Check sheet for the modelled part. Datum: model origin and axes. Units: mm. A direction names the side the tool comes from. Coordinates: 2 decimals unless noted, no trailing zeros. Loops run counter-clockwise (first coordinate to the right, second up) from the corner with the lowest first, then second, coordinate; pieces in that order, holes last. Notation, with made-up numbers: M -10,36 L 45,36 A19 cw 45,65 Z; hole C 1.5,-37.5 d5. An arc over 180 degrees is marked long. Return JSON: item names as keys, results as strings.
from build123d import *

# Parameters (mm, degrees)
BOSS_EXTRUDE1_DEPTH = 145.0848
SKETCH2_R           = 4.50215
SKETCH2_W           = 12.192
SKETCH2_H           = 13.1191
CUT_EXTRUDE1_DEPTH  = 6.35
SKETCH3_W           = 13.1064
SKETCH3_H           = 5.9944
CUT_EXTRUDE2_DEPTH  = 6.35
SKETCH4_W           = 13.0429
SKETCH4_H           = 5.9944
CUT_EXTRUDE3_DEPTH  = 6.35


with BuildPart() as part:
    # Sketch1 → Boss-Extrude1 (new body)
    with BuildSketch(Plane.XY):
        with BuildLine():
            Line((3.110233801, 25.508957203), (61.149233801, 12.137799255))
            ThreePointArc((61.149233801, 12.137799255), (62.566459918, 11.24428163), (63.119, 9.662635945))
            Line((63.119, 9.662635945), (63.119, 2.54))
            ThreePointArc((63.119, 2.54), (62.375051224, 0.743948776), (60.579, 0))
            Line((60.579, 0), (2.54, 0))
            ThreePointArc((2.54, 0), (0.743948776, 0.743948776), (0, 2.54))
            Line((0, 2.54), (0, 23.033793893))
            ThreePointArc((0, 23.033793893), (0.958354315, 25.021253811), (3.110233801, 25.508957203))
        make_face()
    extrude(amount=BOSS_EXTRUDE1_DEPTH)

    # Sketch2 → Cut-Extrude1 (cut)
    with BuildSketch(Plane.XY.offset(145.0848)):
        with Locations((38.989, 8.9154)):
            Circle(SKETCH2_R)
        with Locations((16.9164, 12.65555)):
            Rectangle(SKETCH2_W, SKETCH2_H)
    extrude(amount=-CUT_EXTRUDE1_DEPTH, mode=Mode.SUBTRACT)

    # Sketch3 → Cut-Extrude2 (cut)
    with BuildSketch(Plane.ZY):
        with Locations((31.9532, 10.1854)):
            Rectangle(SKETCH3_W, SKETCH3_H)
        with Locations((53.0352, 10.1854)):
            Rectangle(SKETCH3_W, SKETCH3_H)
        with Locations((74.1172, 10.1854)):
            Rectangle(SKETCH3_W, SKETCH3_H)
        with Locations((95.1992, 10.1854)):
            Rectangle(SKETCH3_W, SKETCH3_H)
        with Locations((116.2812, 10.1854)):
            Rectangle(SKETCH3_W, SKETCH3_H)
    extrude(amount=-CUT_EXTRUDE2_DEPTH, mode=Mode.SUBTRACT)

    # Sketch4 → Cut-Extrude3 (cut)
    with BuildSketch(Plane(origin=(0, 0, 0), x_dir=(-1, 0, 0), z_dir=(0, 0, -1))):
        with Locations((-13.68425, 10.1981)):
            Rectangle(SKETCH4_W, SKETCH4_H)
        with Locations((-35.02025, 10.1981)):
            Rectangle(SKETCH4_W, SKETCH4_H)
    extrude(amount=-CUT_EXTRUDE3_DEPTH, mode=Mode.SUBTRACT)


solid = part.part
1) Draft check along Z on faces 1 (the face through (10.82, 13, 142)), 2 (the face through (25, 10, 0)), 3 (the face through (3, 10, 67.564)). Enter one of: +Z half, -Z half, draft (parallel to the pull), parting line (faces both ways), or undercut.
Answers:
{"face 1": "draft", "face 2": "-Z half", "face 3": "undercut"}
2) Section check A-A on z = 13. Record the cut outline in (x, y).
Answers:
{"outline": "M 0,2.54 A2.54 ccw 2.54,0 L 60.58,0 A2.54 ccw 63.12,2.54 L 63.12,9.66 A2.54 ccw 61.15,12.14 L 3.11,25.51 A2.54 ccw 0,23.03 Z"}
3) Scan lines: line 1 along Y through (x, z) = (3.5, 24); line 2 along X through (y, z) = (7.25, 99); line 3 along X through (y, z) = (5, 139.5). Record each from-to range of solid material in increasing order. Write a range as [from, to].
Answers:
{"line 1": "[0, 25.42]", "line 2": "[6.35, 63.12]", "line 3": "[0, 36.77], [41.21, 63.12]"}
4) Section check C-C on x = 13. Record the cut outline in (y, z).
Answers:
{"outline": "M 0,0 L 7.2,0 L 7.2,6.35 L 13.2,6.35 L 13.2,0 L 23.23,0 L 23.23,145.08 L 19.22,145.08 L 19.22,138.73 L 6.1,138.73 L 6.1,145.08 L 0,145.08 Z"}
5) Section check B-B on y = 14.75. Record the cut outline in (x, z).
Answers:
{"outline": "M 0,0 L 49.81,0 L 49.81,145.08 L 23.01,145.08 L 23.01,138.73 L 10.82,138.73 L 10.82,145.08 L 0,145.08 Z"}
6) Go/stop test with flat-tipped pins: pin 1 Ø5 at (x, z) = (4, 52.5) entering from +Y; pin 2 Ø3 at (x, z) = (4.5, 93) entering from +Y; pin 3 Ø3 at (y, z) = (11, 76.5) entering from -X. Record where each tip stops, or that it passes through.
Answers:
{"pin 1": "y = 25.57", "pin 2": "y = 25.53", "pin 3": "x = 6.35"}
7) Set-up check for faces 4 (the face through (3, 7.188, 74)), 5 (the face through (23.012, 13, 142)), 6 (the face through (14, 13.195, 3)): record each of +Z, -Z, +X, -X, +Y, -Y from which the full face is reachable in a straight line by a thin tool's end or side.
Answers:
{"face 4": "-X", "face 5": "+Z", "face 6": "-Z"}
8) Section check D-D on z = 35. Record the cut outline in (x, y), then the cut area to 3 significant figures.
Answers:
{"outline": "M 0,2.54 A2.54 ccw 2.54,0 L 60.58,0 A2.54 ccw 63.12,2.54 L 63.12,9.66 A2.54 ccw 61.15,12.14 L 3.11,25.51 A2.54 ccw 0,23.03 L 0,13.18 L 6.35,13.18 L 6.35,7.19 L 0,7.19 Z", "area": "1,150 mm²"}
